Check sheet for the modelled part. Datum: model origin and axes. Units: mm. Give positions to 0.01 mm unless a question says otherwise; leave off trailing zeros. Order: outer loops, then holes, each group sorted by start corner. A loop starts at its lowest first (then second) coordinate and runs counter-clockwise, first axis right, second up. Notation, with made-up numbers: (-33, 52.25) -> (-13, 52.25) arc R30 ccw to (-13, 86.25) -> close; hole circle Ø1 at (53, -40). An arc over 180 degrees is marked (long way). Answer in a Markdown table with one row per item. Add a question column.
(1) Thickness scan on L1, parallel to Z at x = -0.25, y = 1.5; L2, parallel to X at y = 0.5, z = 60; L3, parallel to X at y = 0.25, z = 5. Record the ranges inside material, lowest first. Write a range as [from, to].
(2) Go/stop test with flat-tipped pins: pin 1 (2 mm diameter, centred on y = -2, z = 65.5, fed in from -X); pin 2 (1.5 mm diameter, centred on y = -1, z = 78.5, fed in from +X); pin 3 (2 mm diameter, centred on y = -4.5, z = 28, fed in from -X). Record where each tip stops, or that it passes through.
(3) Cross-section at A-A (x = 0). Record the cut outline in (y, z), then the cut area to 3 significant figures.
(4) Cross-section at B-B (y = 0). Record the cut outline in (x, z), then the cut area to 3 significant figures.
(5) Cross-section at D-D (z = 95). Record the cut outline in (x, y), then the cut area to 3 significant figures.
(6) Cross-section at C-C (z = 5). Record the cut outline in (x, y), then the cut area to 3 significant figures.
Autodesk Inventor part; units mm, degrees
ref_plane "YZ Plane" through (0, 0, 0) normal (1, 0, 0) x (0, 1, 0)
ref_plane "XZ Plane" through (0, 0, 0) normal (0, 1, 0) x (-1, 0, 0)
ref_plane "XY Plane" through (0, 0, 0) normal (0, 0, 1) x (1, 0, 0)
sketch "Sketch1" plane through (0, 0, 0) normal (0, 0, 1) x (1, 0, 0)
  circle A0 centre (0, 0) radius 5.75
  dimension "d0" = 11.5
extrude "Extrusion1" add sketch "Sketch1" along normal blind 108
sketch "Sketch2" plane through (0, 0, 0) normal (0, 1, 0) x (-1, 0, 0)
  circle A0 centre (0, 103) radius 2.5
  line L0 (5.75, 108) -> (-5.75, 108)
  circle A1 centre (0, 5) radius 2.5
  point P0 (0, 0)
  dimension "d3" = 5
  dimension "d7" = 5
  dimension "d8" = 5
  dimension "d9" = 5
extrude "Extrusion2" cut sketch "Sketch2" along normal through all both and the other way through all
properties part number "WA001" material "Stainless Steel"
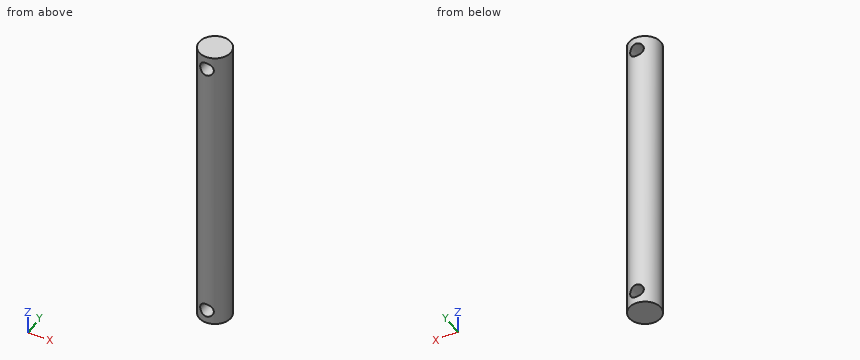
Answer below:
| question | item | result |
|---|---|---|
| 1 | L1 | z = [0, 2.51], [7.49, 100.51], [105.49, 108] |
| 1 | L2 | x = [-5.73, 5.73] |
| 1 | L3 | x = [-5.74, -2.5], [2.5, 5.74] |
| 2 | pin 1 | stops at x = -5.66 |
| 2 | pin 2 | stops at x = 5.74 |
| 2 | pin 3 | stops at x = -4.56 |
| 3 | outline | (-5.75, 0) -> (5.75, 0) -> (5.75, 2.5) -> (-5.75, 2.5) -> close; (-5.75, 7.5) -> (5.75, 7.5) -> (5.75, 100.5) -> (-5.75, 100.5) -> close; (-5.75, 105.5) -> (5.75, 105.5) -> (5.75, 108) -> (-5.75, 108) -> close |
| 3 | area | 1,130 mm² |
| 4 | outline | (-5.75, 0) -> (5.75, 0) -> (5.75, 108) -> (-5.75, 108) -> close; hole circle Ø5 at (0, 5); hole circle Ø5 at (0, 103) |
| 4 | area | 1,200 mm² |
| 5 | outline | circle Ø11.5 at (0, 0) |
| 5 | area | 104 mm² |
| 6 | outline | (-2.5, -5.18) -> (-2.5, 5.18) arc R5.75 ccw to start; (2.5, -5.18) arc R5.75 ccw to (2.5, 5.18) -> close |
| 6 | area | 48.2 mm² |
